Design review of the part shown in the three views and the two pictorial views. Dimensions are in mm from the part's minimum x, y and z. Coordinates: 2 decimals unless noted, no trailing zeros. Loops run counter-clockwise (first coordinate to the right, second up) from the corner with the lowest first, then second, coordinate; pieces in that order, holes last. Notation, with made-up numbers: M 41,86 L 100,86 A5 cw 100,90 Z; hole C 74.25,26 d7. An arc over 180 degrees is marked long. Use one line per item in the form item = value.
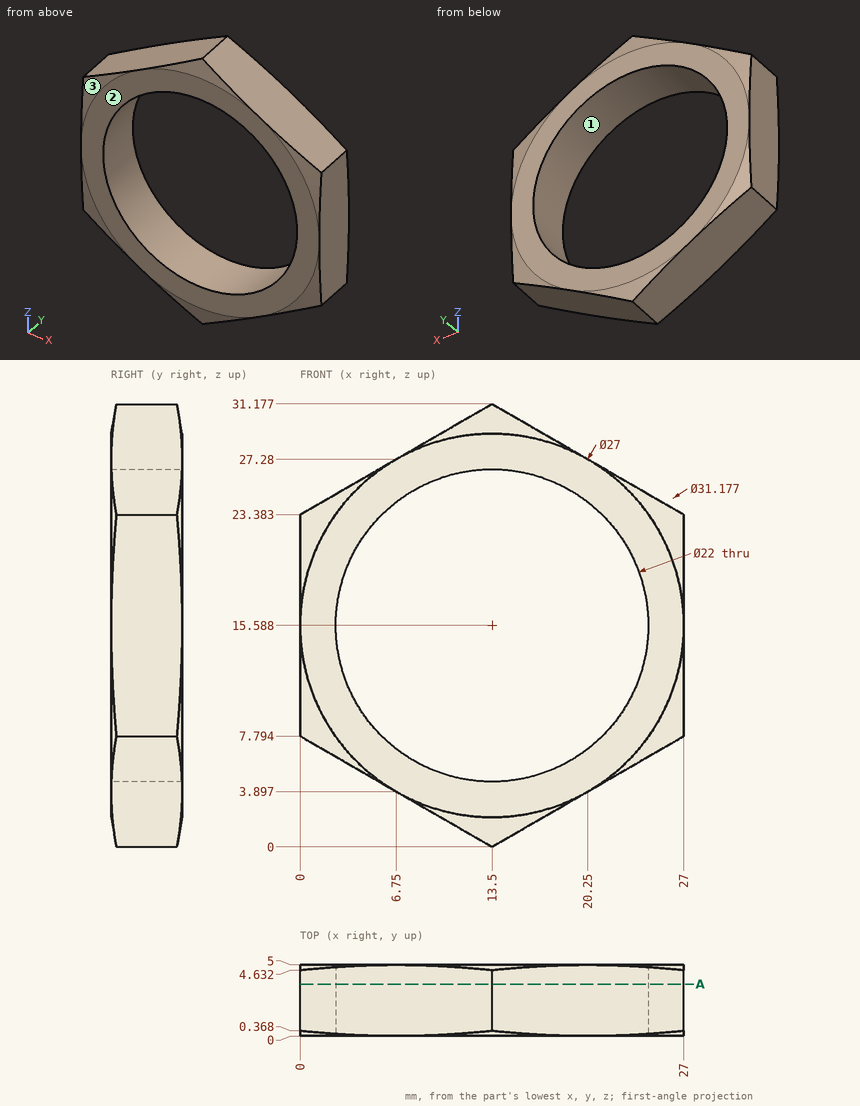
1. Wall thickness on line 1 along X through (y, z) = (3.9, 19); line 2 along Z through (x, y) = (5, 0.4) (1 decimal); line 3 along X through (y, z) = (0.9, 20.5): over which ranges is each line inside the solid? List them lowest first. Write a range as from..to.
Response values:
line_1 = 0..3.04, 23.96..27
line_2 = 4.9..8.6, 22.6..26.3
line_3 = 0..3.66, 23.34..27
2. Add section A-A (y = 3.65). State the section outline as (x, z) points (1 decimal).
Response values:
outline = M 0,7.8 L 13.5,0 L 27,7.8 L 27,23.4 L 13.5,31.2 L 0,23.4 Z; hole C 13.5,15.6 d22
3. Insertion check: P1, Ø2, axis at y = 1.5, z = 4.5, coming from the +X side (1 decimal); P2, Ø3, axis at y = 4, z = 27.5, coming from the -X side (1 decimal); P3, Ø2, axis at x = 20, z = 10.5, coming from the +Y side (3 decimals). Each pin has a flat end and moves straight along its axis. Give the tip position at first contact, or say it passes through.
Response values:
P1 = 23
P2 = 4.5
P3 = through
4. The part is to be moulded in two halves that separate along Z. For the marked faces 1, 2 and 3, say which applies: pulls with the +Z half, pulls with the -Z half, needs draft (parallel to the pull), parting line crosses it, or undercut.
Response values:
face_1 = undercut
face_2 = needs draft
face_3 = pulls with the +Z half
